Build history of the part. All positions in model axes, mm. A direction names the side the tool comes from. Round coordinates to 2 decimals unless told otherwise and drop trailing zeros. Write each loop counter-clockwise with the first axis right and the second up, starting at its lowest first coordinate (ties: lowest second). Pieces come first, ordered by that corner, then holes. Notation, with made-up numbers: (45.5, 47) -> (72.5, 47) arc R21 ccw to (72.5, 86) -> close; hole circle Ø6 at (0, 54.25). An arc over 180 degrees is marked (long way). One line per question, with ' | ' between items.
from build123d import *

# Parameters (mm, degrees)
SKETCH1_W               = 80
SKETCH1_H               = 80
SKETCH1_R               = 3
BOSS_EXTRUDE1_DEPTH     = 100
SKETCH2_W               = 80
SKETCH2_H               = 60
CUT_EXTRUDE1_DEPTH      = 70
SKETCH3_R               = 3
CUT_EXTRUDE2_DEPTH      = 1
CUT_EXTRUDE2_DEPTH_BACK = 81
FILLET1_R               = 10


with BuildPart() as part:
    # Sketch1 → Boss-Extrude1 (new body)
    with BuildSketch(Plane.XY):
        with Locations((40, 40)):
            Rectangle(SKETCH1_W, SKETCH1_H)
        with Locations((40, 40)):
            Circle(SKETCH1_R, mode=Mode.SUBTRACT)
    extrude(amount=BOSS_EXTRUDE1_DEPTH)

    # Sketch2 → Cut-Extrude1 (cut)
    with BuildSketch(Plane.XY.offset(100)):
        with Locations((40, 40)):
            Rectangle(SKETCH2_W, SKETCH2_H)
    extrude(amount=-CUT_EXTRUDE1_DEPTH, mode=Mode.SUBTRACT)

    # Sketch3 → Cut-Extrude2 (cut, two sides)
    with BuildSketch(Plane(origin=(0, 80, 0), x_dir=(1, 0, 0), z_dir=(0, 1, 0))) as cut_extrude2_sk:
        with Locations((40, -65)):
            Circle(SKETCH3_R)
    extrude(amount=CUT_EXTRUDE2_DEPTH, mode=Mode.SUBTRACT)
    extrude(cut_extrude2_sk.sketch, amount=-CUT_EXTRUDE2_DEPTH_BACK, mode=Mode.SUBTRACT)

    # Fillet1
    fillet1_edges = [part.edges().sort_by_distance(p)[0] for p in [
        (80, 5, 100),
        (80, 75, 100),
        (0, 5, 100),
        (0, 75, 100),
    ]]
    fillet(fillet1_edges, radius=FILLET1_R)


solid = part.part
(1) Mould opens along Z. For faces 3 (the flat face through (80, 39, 24)), 4 (the cylindrical face through (2.85, 75.07, 96.99)), 5 (the flat face through (48, 41, 0)), 6 (the cylindrical face through (37.6, 5.1, 66.8)) say: pulls with the +Z half, pulls with the -Z half, needs draft (parallel to the pull), parting line crosses it, or undercut.
Calculated:
face 3: needs draft | face 4: pulls with the +Z half | face 5: pulls with the -Z half | face 6: undercut
(2) Slice it at D-D (x = 51.5). Write the cut outline in (y, z), then the cut area to 3 significant figures.
Calculated:
outline: (0, 0) -> (80, 0) -> (80, 100) -> (70, 100) -> (70, 30) -> (10, 30) -> (10, 100) -> (0, 100) -> close | area: 3,800 mm2
(3) Slice it at A-A (x = 40). Write the cut outline in (y, z), then the cut area to 3 significant figures.
Calculated:
outline: (0, 0) -> (37, 0) -> (37, 30) -> (10, 30) -> (10, 62) -> (0, 62) -> close; (0, 68) -> (10, 68) -> (10, 100) -> (0, 100) -> close; (43, 0) -> (80, 0) -> (80, 62) -> (70, 62) -> (70, 30) -> (43, 30) -> close; (70, 68) -> (80, 68) -> (80, 100) -> (70, 100) -> close | area: 3,500 mm2
(4) Slice it at B-B (z = 40). Write the cut outline in (x, y).
Calculated:
outline: (0, 0) -> (80, 0) -> (80, 10) -> (0, 10) -> close; (0, 70) -> (80, 70) -> (80, 80) -> (0, 80) -> close
(5) Wall check: line 1 (Z direction, x = 40, y = 77); line 2 (X direction, y = 73.5, z = 65); line 3 (Y direction, x = 63, z = 72). Give the ranges that are in metal, low to high. Write a range as from..to.
Calculated:
line 1: 0..62, 68..100 | line 2: 0..37, 43..80 | line 3: 0..10, 70..80
(6) Slice it at C-C (y = 40). Write the cut outline in (x, z), then the cut area to 3 significant figures.
Calculated:
outline: (0, 0) -> (37, 0) -> (37, 30) -> (0, 30) -> close; (43, 0) -> (80, 0) -> (80, 30) -> (43, 30) -> close | area: 2,220 mm2
(7) Drop a flat-ended pin along its axis: pin 1 (12 mm diameter, centred on x = 70.5, y = 18, fed in from +Z). Give the stop position or say it passes through.
Calculated:
pin 1: z = 30
(8) 3-axis set-ups, long thin cutter, end or side, ignore diameter. For faces 1 (the flat face through (39, 47, 30)), 2 (the cylindrical face through (2.85, 5.07, 96.99)): which of +Z, -Z, +X, -X, +Y, -Y reach the whole face in a straight line?
Calculated:
face 1: +Z, +X, -X | face 2: +Z, -X, +Y, -Y
